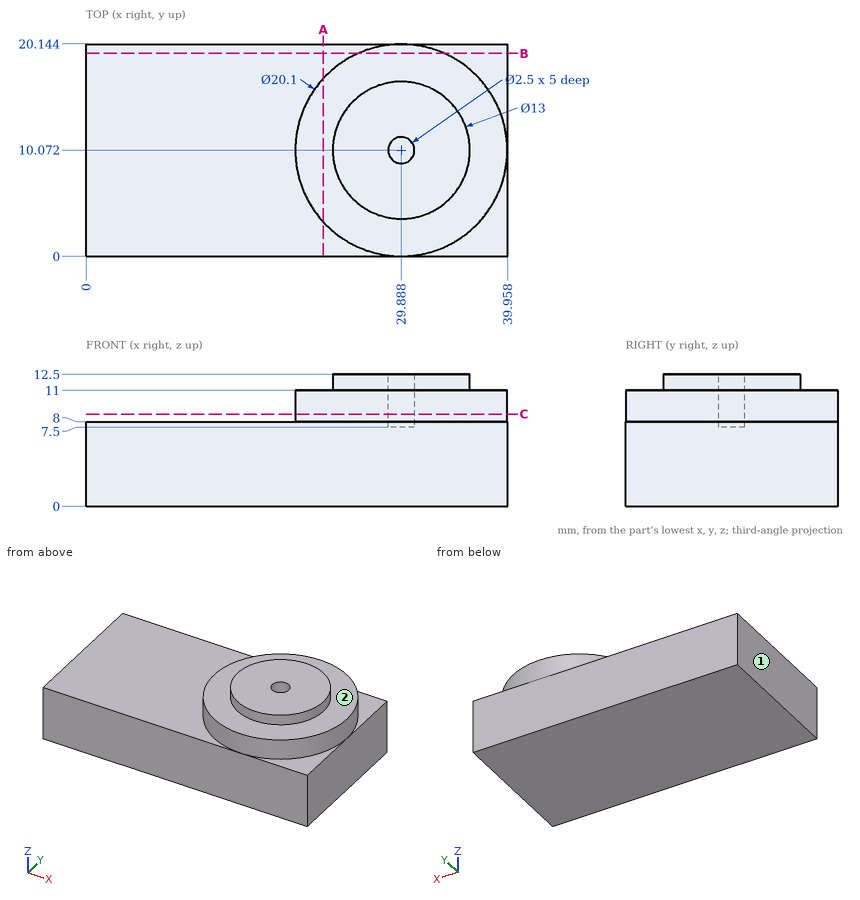
For this review, use the dimensioned drawing (mm, ordinates from the lowest corner) and the shaded views. A direction names the side the tool comes from. Give positions to 0.01 mm unless a question says otherwise; leave off trailing zeros. Order: outer loops, then holes, each group sorted by start corner. A loop starts at its lowest first (then second) coordinate and runs counter-clockwise, first axis right, second up. Notation, with made-up numbers: (20, 42.5) -> (37, 42.5) arc R18 ccw to (37, 61.5) -> close; hole circle Ø3 at (14, 28.25). An arc over 180 degrees is marked (long way). Write item = value, one per line. Start each with the question number.
(1) Take a section at B-B (y = 19.25). Write out the cut boundary in (x, z) (1 decimal).
(2) For L1, parallel to Z at x = 7.5, y = 11; L2, parallel to Y at x = 30, z = 12; L3, parallel to Z at x = 25, y = 5.5, list the stretches that pass through material, from the lowest coordinate up. Write a range as from..to.
(3) Take a section at C-C (z = 8.75). Write out the cut boundary in (x, y).
(4) Take a section at A-A (x = 22.5). Write out the cut boundary in (y, z) (1 decimal).
(5) Tool access review of the marked faces 1 and 2: name each direction out of +Z, -Z, +X, -X, +Y, -Y from which nothing blocks a thin tool from reaching the whole face with its end or side.
Returned:
q1.outline = (0, 0) -> (40, 0) -> (40, 8) -> (34, 8) -> (34, 11) -> (25.8, 11) -> (25.8, 8) -> (0, 8) -> close
q2.L1 = 0..8
q2.L2 = 3.57..8.83, 11.32..16.57
q2.L3 = 0..11
q3.outline = circle Ø20.1 at (29.89, 10.07); hole circle Ø2.5 at (29.89, 10.07)
q4.outline = (0, 0) -> (20.1, 0) -> (20.1, 8) -> (16.9, 8) -> (16.9, 11) -> (3.3, 11) -> (3.3, 8) -> (0, 8) -> close
q5.face_1 = +Z, -Z, -X, +Y, -Y
q5.face_2 = +Z
